Geometry: final body of the model. Coordinates: model frame, mm. A direction names the side the tool comes from. Give positions to 0.01 mm unless a question says otherwise; leave off trailing zeros. Order: outer loops, then holes, each group sorted by start corner. A loop starts at its lowest first (then second) coordinate and runs counter-clockwise, first axis right, second up. Notation, with made-up numbers: (-7.5, -4) - (15.5, -4) arc R15 ccw to (15.5, 23) - close; hole circle Ø9 at (80, -2). An arc over 180 degrees is marked (long way). Put each result on its own line as item: value. Start each with the question number.
1. Section B-B on x = 0. Return the cut outline in (y, z).
2. Ray query, line 1 along X through (y, z) = (-1, -11); line 2 along X through (y, z) = (7, -54); line 3 along Z through (x, y) = (-59, -1). Return the intervals inside material, ascending. Write a range as from..to.
3. Set-up query: faces 1 (the flat face through (79, -15, 0)), 2 (the flat face through (49, -19.05, 6)), 3 (the flat face through (-50, -19.05, 6)), 4 (the flat face through (-79, -14, 0)), 5 (the flat face through (-79, 15, 0)). Return all of +Z, -Z, +X, -X, +Y, -Y with unobstructed straight access to the full face (end or side cutting, diameter ignored); none if empty.
4. Section D-D on z = 25. Return the cut outline in (x, y), plus the area to 3 significant figures.
5. Section C-C on y = 10. Return the cut outline in (x, z), plus the area to 3 significant figures.
6. Mould query, pull axis X, two halves, no side actions, for faces 6 (the flat face through (-64, 0, -76.2)), 7 (the flat face through (-82.55, 0, 6)), 8 (the flat face through (-15, 17, 0)), 9 (the cylindrical face through (15.12, 11.59, -37.57)). Classes: pulls with the +X half, pulls with the -X half, needs draft (parallel to the pull), parting line crosses it, or undercut.
7. First-contact query: P1, Ø1, axis at x = 37, y = 4.5, coming from the -Z side; P2, Ø5, axis at x = -35, y = -16.5, coming from the +Z side; P3, Ø14, axis at x = 48.5, z = 9.5, coming from the -Y side. Flat tips, straight axial feed; report the tip coordinate or a pass-through.
8. Section A-A on z = -23. Return the cut outline in (x, y).
from build123d import *

# Parameters (mm, degrees)
F1_DEPTH = 101.6
F2_DEPTH = 12.7
F4_DEPTH = 76.2


with BuildPart() as f1:
    # F0 (on Top) → F1 (new body)
    with BuildSketch(Plane.XY):
        with BuildLine():
            ThreePointArc((-16.8005208253, -19.05), (0, -25.4), (16.8005208253, -19.05))
            Line((16.8005208253, -19.05), (-16.8005208253, -19.05))
        make_face()
        with BuildLine():
            ThreePointArc((25.4, 0), (23.1505208253, 10.4505208253), (16.8005208253, 19.05))
            Line((16.8005208253, 19.05), (-16.8005208253, 19.05))
            ThreePointArc((-16.8005208253, 19.05), (-25.4, 0), (-16.8005208253, -19.05))
            Line((-16.8005208253, -19.05), (16.8005208253, -19.05))
            ThreePointArc((16.8005208253, -19.05), (23.1505208253, -10.4505208253), (25.4, 0))
        make_face()
        with BuildLine():
            Line((-16.8005208253, 19.05), (16.8005208253, 19.05))
            ThreePointArc((16.8005208253, 19.05), (0, 25.4), (-16.8005208253, 19.05))
        make_face()
    extrude(amount=F1_DEPTH)

    # F0 (on Top) → F2 (join)
    with BuildSketch(Plane.XY):
        with BuildLine():
            Line((82.55, -19.05), (82.55, 19.05))
            Line((82.55, 19.05), (16.8005208253, 19.05))
            ThreePointArc((16.8005208253, 19.05), (23.1505208253, 10.4505208253), (25.4, 0))
            ThreePointArc((25.4, 0), (23.1505208253, -10.4505208253), (16.8005208253, -19.05))
            Line((16.8005208253, -19.05), (82.55, -19.05))
        make_face()
        with BuildLine():
            ThreePointArc((25.4, 0), (23.1505208253, 10.4505208253), (16.8005208253, 19.05))
            Line((16.8005208253, 19.05), (-16.8005208253, 19.05))
            ThreePointArc((-16.8005208253, 19.05), (-25.4, 0), (-16.8005208253, -19.05))
            Line((-16.8005208253, -19.05), (16.8005208253, -19.05))
            ThreePointArc((16.8005208253, -19.05), (23.1505208253, -10.4505208253), (25.4, 0))
        make_face()
        with BuildLine():
            Line((-16.8005208253, 19.05), (16.8005208253, 19.05))
            ThreePointArc((16.8005208253, 19.05), (0, 25.4), (-16.8005208253, 19.05))
        make_face()
        with BuildLine():
            ThreePointArc((-16.8005208253, -19.05), (-25.4, 0), (-16.8005208253, 19.05))
            Line((-16.8005208253, 19.05), (-82.55, 19.05))
            Line((-82.55, 19.05), (-82.55, -19.05))
            Line((-82.55, -19.05), (-16.8005208253, -19.05))
        make_face()
        with BuildLine():
            ThreePointArc((-16.8005208253, -19.05), (0, -25.4), (16.8005208253, -19.05))
            Line((16.8005208253, -19.05), (-16.8005208253, -19.05))
        make_face()
    extrude(amount=F2_DEPTH)

    # F3 (on Top) → F4 (join)
    with BuildSketch(Plane.XY):
        with BuildLine():
            Line((0, 0), (19.05, 0))
            ThreePointArc((19.05, 0), (0, 19.05), (-19.05, 0))
            Line((-19.05, 0), (0, 0))
        make_face()
        with BuildLine():
            ThreePointArc((-82.55, 0), (-63.5, -19.05), (-44.45, 0))
            Line((-44.45, 0), (-63.5, 0))
            Line((-63.5, 0), (-82.55, 0))
        make_face()
        with BuildLine():
            Line((-63.5, 0), (-44.45, 0))
            ThreePointArc((-44.45, 0), (-63.5, 19.05), (-82.55, 0))
            Line((-82.55, 0), (-63.5, 0))
        make_face()
        with BuildLine():
            ThreePointArc((-19.05, 0), (0, -19.05), (19.05, 0))
            Line((19.05, 0), (0, 0))
            Line((0, 0), (-19.05, 0))
        make_face()
        with BuildLine():
            ThreePointArc((82.55, 0), (63.5, 19.05), (44.45, 0))
            Line((44.45, 0), (63.5, 0))
            Line((63.5, 0), (82.55, 0))
        make_face()
        with BuildLine():
            Line((63.5, 0), (44.45, 0))
            ThreePointArc((44.45, 0), (63.5, -19.05), (82.55, 0))
            Line((82.55, 0), (63.5, 0))
        make_face()
    extrude(amount=-F4_DEPTH)


solid = f1.part
Resolved:
1. outline: (-25.4, 0) - (-19.05, 0) - (-19.05, -76.2) - (19.05, -76.2) - (19.05, 0) - (25.4, 0) - (25.4, 101.6) - (-25.4, 101.6) - close
2. line 1: -82.52..-44.48, -19.02..19.02, 44.48..82.52
2. line 2: -81.22..-45.78, -17.72..17.72, 45.78..81.22
2. line 3: -76.2..12.7
3. face 1: -Z, +X, -Y
3. face 2: +Z, -Z, +X, -Y
3. face 3: +Z, -Z, -X, -Y
3. face 4: -Z, -X, -Y
3. face 5: -Z, -X, +Y
4. outline: circle Ø50.8 at (0, 0)
4. area: 2,030 mm^2
5. outline: (-82.55, 0) - (-79.71, 0) - (-79.71, -76.2) - (-47.29, -76.2) - (-47.29, 0) - (-16.21, 0) - (-16.21, -76.2) - (16.21, -76.2) - (16.21, 0) - (47.29, 0) - (47.29, -76.2) - (79.71, -76.2) - (79.71, 0) - (82.55, 0) - (82.55, 12.7) - (23.35, 12.7) - (23.35, 101.6) - (-23.35, 101.6) - (-23.35, 12.7) - (-82.55, 12.7) - close
5. area: 13,700 mm^2
6. face 6: needs draft
6. face 7: pulls with the -X half
6. face 8: undercut
6. face 9: undercut
7. P1: z = 0
7. P2: z = 12.7
7. P3: y = -19.05
8. outline: circle Ø38.1 at (-63.5, 0); circle Ø38.1 at (0, 0); circle Ø38.1 at (63.5, 0)
